The listing builds one solid part. Answer for the finished solid, in the listing's coordinates (mm). A direction names the side the tool comes from. Round coordinates to 2 decimals unless told otherwise and drop trailing zeros. Write each loop counter-clockwise with the first axis right and the second up, starting at its lowest first coordinate (ties: lowest second). Pieces come first, ordered by that corner, then holes. Notation, with made-up numbers: (18, 64) - (35, 64) arc R23 cw to (35, 96) - close; hole circle Ø4 at (-34, -0.5). An arc over 180 degrees is marked (long way). Return JSON: item names as keys, results as strings. Group by question number.
from build123d import *

# Parameters (mm, degrees)
EXTRUDE_1_DEPTH     = 25
SKETCH_4_R          = 2.5
CUT_EXTRUDE_1_DEPTH = 69.766316506
SKETCH_5_R          = 2.5
CUT_EXTRUDE_2_DEPTH = 69.766316506


with BuildPart() as part:
    # 草圖1 → 填料-伸長1 (new body)
    with BuildSketch(Plane.XY):
        with BuildLine():
            Line((0, 0), (52.305552833, 0))
            Line((52.305552833, 0), (52.305552833, 2.314523209))
            Line((52.305552833, 2.314523209), (32.501449094, 2.314523209))
            ThreePointArc((32.501449094, 2.314523209), (30.103466052, 12.469263913), (24.618610108, 21.345379996))
            Line((24.618610108, 21.345379996), (38.622226158, 35.348996046))
            Line((38.622226158, 35.348996046), (36.985611102, 36.985611102))
            Line((36.985611102, 36.985611102), (0, 0))
        make_face()
        with BuildLine():
            Line((29.470981811, 2.314523209), (13.368711302, 2.314523209))
            Line((13.368711302, 2.314523209), (28.312069292, 8.504264755))
            ThreePointArc((28.312069292, 8.504264755), (29.056814584, 5.44034124), (29.470981811, 2.314523209))
        make_face(mode=Mode.SUBTRACT)
        with BuildLine():
            Line((11.089721473, 7.816491361), (26.033079463, 14.006232908))
            ThreePointArc((26.033079463, 14.006232908), (24.393172815, 16.69936845), (22.475746143, 19.202516031))
            Line((22.475746143, 19.202516031), (11.089721473, 7.816491361))
        make_face(mode=Mode.SUBTRACT)
    extrude(amount=EXTRUDE_1_DEPTH)

    # 草圖4 → 除料-伸長1 (cut, through all)
    with BuildSketch(Plane.XZ):
        with Locations((42.305552833, 12.5)):
            Circle(SKETCH_4_R)
    extrude(amount=-CUT_EXTRUDE_1_DEPTH, mode=Mode.SUBTRACT)

    # 草圖5 → 除料-伸長2 (cut, through all)
    with BuildSketch(Plane(origin=(0, 0, 0), x_dir=(0, 0, 1), z_dir=(-0.7071067811865479, 0.7071067811865472, 0))):
        with Locations(Location((12.5, 42.305552833, 0), (0, 0, 270))):
            Circle(SKETCH_5_R)
    extrude(amount=-CUT_EXTRUDE_2_DEPTH, mode=Mode.SUBTRACT)


solid = part.part
(1) Find section B-B (y = 5). Write down the section's boundary in (x, z), plus the area to 3 significant figures.
(2) Find section C-C (x = 23.5). Write down the section's boundary in (y, z), plus the area to 3 significant figures.
(3) Flat-ended cylindrical pins translate along their axes: pin 1 (10 mm diameter, centred on x = 44, z = 12, fed in from +Y); pin 2 (10 mm diameter, centred on y = 21, z = 21.5, fed in from +X); pin 3 (4.5 mm diameter, centred on x = 42.31, z = 12.5, fed in from -Y); pin 4 (6 mm diameter, centred on y = 32.5, z = 17.5, fed in from +X). Find the tip coordinate at first contact, or state that the pin passes through.
(4) Consider line 1 (Y direction, x = 24.5, z = 3.25); line 2 (Y direction, x = 19.5, z = 7.5); line 3 (Y direction, x = 34, z = 23). Determine where each line is inside the solid, lowest interval first.
(5) Find section A-A (z = 18.5). Write down the section's boundary in (x, y).
(6) Find section D-D (z = 12.5). Write down the section's boundary in (x, y).
(7) For faces 1 (the cylindrical face through (29.05, 5.48, 12.32)), 2 (the cylindrical face through (44.615, 1.141, 11.542)), 3 (the cylindrical face through (30.16, 12.33, 12.32)), determine the directions among +Z, -Z, +X, -X, +Y, -Y from which every point of the face is accessible in a straight line to the end or side of a thin tool.
(8) Determine the mould class of faces 4 (the flat face through (19, 19, 12)), 5 (the flat face through (18.46, 10.87, 12.32)), 6 (the flat face through (16.862, 13.589, 12.325)), 7 (the flat face through (22, 8, 25)) for opening direction X: +X half, -X half, draft (parallel to the pull), parting line (faces both ways), or undercut.
Check sheet entries:
{
 "1": {"outline": "(5, 0) - (19.85, 0) - (19.85, 25) - (5, 25) - close; (29.14, 0) - (32.2, 0) - (32.2, 25) - (29.14, 25) - close", "area": "448 mm^2"},
 "2": {"outline": "(0, 0) - (2.31, 0) - (2.31, 25) - (0, 25) - close; (6.51, 0) - (12.96, 0) - (12.96, 25) - (6.51, 25) - close; (17.93, 0) - (23.5, 0) - (23.5, 25) - (17.93, 25) - close", "area": "358 mm^2"},
 "3": {"pin 1": "stops at y = 2.31", "pin 2": "stops at x = 29.27", "pin 3": "passes through", "pin 4": "stops at x = 38.62"},
 "4": {"line 1": "y = 0 to 2.31, 6.93 to 13.37, 16.54 to 24.5", "line 2": "y = 0 to 2.31, 4.85 to 11.3, 16.23 to 19.5", "line 3": "y = 0 to 2.31, 30.73 to 34"},
 "5": {"outline": "(0, 0) - (52.31, 0) - (52.31, 2.31) - (32.5, 2.31) arc R32.58 ccw to (24.62, 21.35) - (38.62, 35.35) - (36.99, 36.99) - close; hole (11.09, 7.82) - (26.03, 14.01) arc R29.56 ccw to (22.48, 19.2) - close; hole (13.37, 2.31) - (29.47, 2.31) arc R29.56 ccw to (28.31, 8.5) - close"},
 "6": {"outline": "(0, 0) - (39.81, 0) - (39.81, 2.31) - (32.5, 2.31) arc R32.58 ccw to (24.62, 21.35) - (29.78, 26.51) - (28.15, 28.15) - close; (31.68, 31.68) - (33.32, 30.05) - (38.62, 35.35) - (36.99, 36.99) - close; (44.81, 0) - (52.31, 0) - (52.31, 2.31) - (44.81, 2.31) - close; hole (11.09, 7.82) - (26.03, 14.01) arc R29.56 ccw to (22.48, 19.2) - close; hole (13.37, 2.31) - (29.47, 2.31) arc R29.56 ccw to (28.31, 8.5) - close"},
 "7": {"face 1": "+Z, -Z", "face 2": "+Y, -Y", "face 3": "+Z, -Z, +X"},
 "8": {"face 4": "-X half", "face 5": "undercut", "face 6": "undercut", "face 7": "draft"}
}
